Geometry check sheet. Reference: the model listing, model coordinates, mm. Coordinates: 2 decimals unless noted, no trailing zeros. Loops run counter-clockwise (first coordinate to the right, second up) from the corner with the lowest first, then second, coordinate; pieces in that order, holes last.
from build123d import *

# Parameters (mm, degrees)
MASTER_R            = 79.375
MASTER_R_2          = 1.984375
MASTER_R_3          = 1.143
MASTER_R_4          = 1.0414
MASTER_R_5          = 1.6002
BOSS_EXTRUDE1_DEPTH = 6.35
SKETCH11_R          = 1.143
BOSS_EXTRUDE3_DEPTH = 7.62
SKETCH13_W          = 13.5382
SKETCH13_H          = 5.08
CUT_EXTRUDE1_DEPTH  = 173.000625072


with BuildPart() as part:
    # Master → Boss-Extrude1 (new body)
    with BuildSketch(Plane.XY):
        Circle(MASTER_R)
        with Locations((-28.39, -56.515)):
            Circle(MASTER_R_2, mode=Mode.SUBTRACT)
        with BuildLine():
            ThreePointArc((-73.025, 20.32), (-68.2625, 25.0825), (-63.5, 20.32))
            Line((-63.5, 20.32), (-63.5, -20.32))
            ThreePointArc((-63.5, -20.32), (-68.2625, -25.0825), (-73.025, -20.32))
            Line((-73.025, -20.32), (-73.025, 20.32))
        make_face(mode=Mode.SUBTRACT)
        with Locations((-46.6725, -8.89)):
            Circle(MASTER_R_3, mode=Mode.SUBTRACT)
        with Locations((-28.39, -14.615)):
            Circle(MASTER_R_2, mode=Mode.SUBTRACT)
        with Locations((37.71, -56.515)):
            Circle(MASTER_R_2, mode=Mode.SUBTRACT)
        with Locations((37.71, -14.615)):
            Circle(MASTER_R_2, mode=Mode.SUBTRACT)
        with Locations((46.6725, -8.89)):
            Circle(MASTER_R_3, mode=Mode.SUBTRACT)
        with BuildLine():
            Line((63.5, -20.32), (63.5, 20.32))
            ThreePointArc((63.5, 20.32), (68.2625, 25.0825), (73.025, 20.32))
            Line((73.025, 20.32), (73.025, -20.32))
            ThreePointArc((73.025, -20.32), (68.2625, -25.0825), (63.5, -20.32))
        make_face(mode=Mode.SUBTRACT)
        with Locations((-46.6725, 8.89)):
            Circle(MASTER_R_3, mode=Mode.SUBTRACT)
        with BuildLine():
            Line((-43.949373457, 43.949373457), (-53.531306738, 34.367440175))
            Line((-53.531306738, 34.367440175), (-60.200586388, 41.036719826))
            Line((-60.200586388, 41.036719826), (-59.13351137, 42.103794844))
            ThreePointArc((-59.13351137, 42.103794844), (-58.829657849, 42.790920417), (-58.142532276, 43.094773938))
            Line((-58.142532276, 43.094773938), (-50.618653107, 50.618653107))
            Line((-50.618653107, 50.618653107), (-43.949373457, 43.949373457))
        make_face(mode=Mode.SUBTRACT)
        with Locations((-37.492569305, 53.531306738)):
            Circle(MASTER_R_4, mode=Mode.SUBTRACT)
        with Locations((-18.478499634, 60.3123)):
            Circle(MASTER_R_5, mode=Mode.SUBTRACT)
        with Locations((46.6725, 8.89)):
            Circle(MASTER_R_3, mode=Mode.SUBTRACT)
        with Locations((53.531306738, 37.492569305)):
            Circle(MASTER_R_4, mode=Mode.SUBTRACT)
        with Locations((18.478500366, 60.3123)):
            Circle(MASTER_R_5, mode=Mode.SUBTRACT)
        with BuildLine():
            Line((43.949373457, 43.949373457), (34.367440175, 53.531306738))
            Line((34.367440175, 53.531306738), (41.036719826, 60.200586388))
            Line((41.036719826, 60.200586388), (42.103794844, 59.13351137))
            ThreePointArc((42.103794844, 59.13351137), (42.790920417, 58.829657849), (43.094773938, 58.142532276))
            Line((43.094773938, 58.142532276), (50.618653107, 50.618653107))
            Line((50.618653107, 50.618653107), (43.949373457, 43.949373457))
        make_face(mode=Mode.SUBTRACT)
    extrude(amount=BOSS_EXTRUDE1_DEPTH)

    # Sketch11 → Boss-Extrude3 (add)
    # profile 1 of 2: a face of its own
    with BuildSketch(Plane.XY):
        with BuildLine():
            Line((6.7691, 67.5132), (-6.7691, 67.5132))
            ThreePointArc((-6.7691, 67.5132), (-9.525, 70.2691), (-6.7691, 73.025))
            Line((-6.7691, 73.025), (6.7691, 73.025))
            ThreePointArc((6.7691, 73.025), (9.525, 70.2691), (6.7691, 67.5132))
        make_face()
        with Locations((-6.7691, 70.2691)):
            Circle(SKETCH11_R, mode=Mode.SUBTRACT)
        with Locations((6.7691, 70.2691)):
            Circle(SKETCH11_R, mode=Mode.SUBTRACT)
    # profile 2 of 2: a face of its own
    with BuildSketch(Plane.XY):
        with BuildLine():
            Line((6.7691, -67.5132), (-6.7691, -67.5132))
            ThreePointArc((-6.7691, -67.5132), (-9.525, -70.2691), (-6.7691, -73.025))
            Line((-6.7691, -73.025), (6.7691, -73.025))
            ThreePointArc((6.7691, -73.025), (9.525, -70.2691), (6.7691, -67.5132))
        make_face()
        with Locations((6.7691, -70.2691)):
            Circle(SKETCH11_R, mode=Mode.SUBTRACT)
        with Locations((-6.7691, -70.2691)):
            Circle(SKETCH11_R, mode=Mode.SUBTRACT)
    extrude(amount=-BOSS_EXTRUDE3_DEPTH)

    # Sketch13 → Cut-Extrude1 (cut, through all)
    with BuildSketch(Plane(origin=(0, 73.025, 0), x_dir=(1, 0, 0), z_dir=(0, 1, 0))):
        with Locations((0, 2.54)):
            Rectangle(SKETCH13_W, SKETCH13_H)
    extrude(amount=-CUT_EXTRUDE1_DEPTH, mode=Mode.SUBTRACT)


solid = part.part
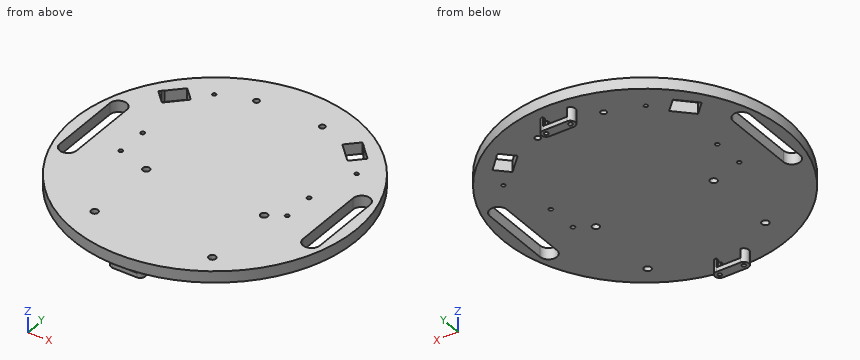
(1) Scan lines: L1, parallel to X at y = 2.5, z = 3.25 (3 decimals); L2, parallel to X at y = -55, z = 5; L3, parallel to Z at x = 10, y = 32. Record each from-to range of solid material in increasing order.
Findings:
L1: x = -79.336 to -73.025, -63.5 to 63.5, 73.025 to 79.336
L2: x = -57.23 to -29.67, -27.11 to 36.43, 38.99 to 57.23
L3: z = 0 to 6.35
(2) Sectioned sample at D-D on y = -2. Record the cut outline in (x, z) (3 decimals), and give its area (3 significant figures).
Findings:
outline: (-79.35, 0) - (-73.025, 0) - (-73.025, 6.35) - (-79.35, 6.35) - close; (-63.5, 0) - (63.5, 0) - (63.5, 6.35) - (-63.5, 6.35) - close; (73.025, 0) - (79.35, 0) - (79.35, 6.35) - (73.025, 6.35) - close
area: 887 mm2
(3) Sectioned sample at C-C on x = -55.5. Record the cut outline in (y, z), and give its area (3 significant figures).
Findings:
outline: (-56.75, 0) - (36.34, 0) - (36.34, 6.35) - (-56.75, 6.35) - close; (45.74, 0) - (56.75, 0) - (56.75, 6.35) - (45.74, 6.35) - close
area: 661 mm2
(4) Sectioned sample at A-A on x = 0. Record the cut outline in (y, z) (3 decimals), and give its area (3 significant figures).
Findings:
outline: (-79.375, 0) - (79.375, 0) - (79.375, 6.35) - (-79.375, 6.35) - close; (-73.025, -7.62) - (-67.513, -7.62) - (-67.513, -5.08) - (-73.025, -5.08) - close; (67.513, -7.62) - (73.025, -7.62) - (73.025, -5.08) - (67.513, -5.08) - close
area: 1,040 mm2
(5) Gauge pin test, flat ends, axial feed: pin 1 Ø3 at (x, z) = (1.5, -6.5) entering from +Y (3 decimals); pin 2 Ø0.5 at (y, z) = (-68.5, -1.5) entering from +X; pin 3 Ø2.5 at (x, y) = (46.67, 8.89) entering from -Z; pin 4 Ø3 at (x, y) = (-6.77, 70.27) entering from -Z. Record the tip position at first contact, or that the pin passes through.
Findings:
pin 1: stops at y = 73.025
pin 2: stops at x = 9.07
pin 3: stops at z = 0
pin 4: stops at z = -7.62
(6) Sectioned sample at B-B on z = 2.75. State how many separate pieces and enclosed holes the cut face has, and give its area (3 significant figures).
Findings:
separate pieces: 1
enclosed holes: 16
area: 18,500 mm2
